```python
from build123d import *

# Parameters (mm, degrees)
F0_W     = 200
F0_H     = 25
F0_H_2   = 5
F1_DEPTH = 5
F2_DEPTH = 13.2
F3_SIZE  = 0.6


with BuildPart() as f1:
    # F0 (on Top) → F1 (new body)
    with BuildSketch(Plane.XY):
        with Locations((100, 12.5)):
            Rectangle(F0_W, F0_H)
        with Locations((100, -2.5)):
            Rectangle(F0_W, F0_H_2)
    extrude(amount=F1_DEPTH)

    # F0 (on Top) → F2 (join)
    with BuildSketch(Plane.XY):
        with Locations((100, -2.5)):
            Rectangle(F0_W, F0_H_2)
    extrude(amount=F2_DEPTH)

    # F3
    f3_edges = [f1.edges().sort_by_distance(p)[0] for p in [
        (100, 25, 5),
        (200, 12.5, 5),
        (200, 25, 2.5),
        (200, 10, 0),
        (200, -5, 6.6),
        (200, -2.5, 13.2),
        (200, 0, 9.1),
        (0, 25, 2.5),
        (100, 25, 0),
        (0, 10, 0),
        (0, 12.5, 5),
        (0, 0, 9.1),
        (0, -2.5, 13.2),
        (0, -5, 6.6),
        (100, 0, 13.2),
        (100, -5, 13.2),
        (100, -5, 0),
    ]]
    chamfer(f3_edges, length=F3_SIZE)


solid = f1.part
```
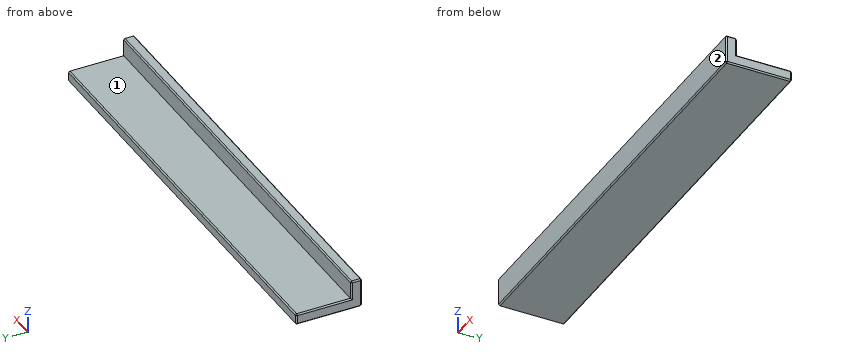
CAD build for the part. Positions are in the model's coordinates, mm. Face numbers are marked on the shaded views. A direction names the side the tool comes from. Round coordinates to 2 decimals unless told otherwise and drop trailing zeros. Order: outer loops, then holes, each group sorted by start corner. A loop starts at its lowest first (then second) coordinate and runs counter-clockwise, first axis right, second up.
Q1. Drop a flat-ended pin along its axis: pin 1 (6 mm diameter, centred on x = 121.5, z = 10, fed in from +Y). Give the stop position or say it passes through.
Q2. Which spindle directions (+Z, -Z, +X, -X, +Y, -Y) get a long thin tool onto all of the face, cutting with end or side? Do the marked faces 1 and 2. Say none if no direction does.
Q3. Slice it at C-C (x = 111). Write the cut outline in (y, z).
Q4. Slice it at B-B (z = 7.5). Write the cut outline in (x, y).
Q5. Slice it at A-A (y = 14.5). Write the cut outline in (x, z).
Q6. Wall check: L1, parallel to Z at x = 158, y = 5.5; L2, parallel to Y at x = 74.5, z = 5.5; L3, parallel to Y at x = 124, z = 4.5. Give the ranges that are in metal, low to high.
Results below:
1. pin 1: stops at y = 0
2. face 1: +Z, +X, -X, +Y
2. face 2: +Z, -Z, +X, -X, -Y
3. outline: (-5, 0.6) - (-4.4, 0) - (24.4, 0) - (25, 0.6) - (25, 4.4) - (24.4, 5) - (0, 5) - (0, 12.6) - (-0.6, 13.2) - (-4.4, 13.2) - (-5, 12.6) - close
4. outline: (0, -4.4) - (0.6, -5) - (199.4, -5) - (200, -4.4) - (200, -0.6) - (199.4, 0) - (0.6, 0) - (0, -0.6) - close
5. outline: (0, 0.6) - (0.6, 0) - (199.4, 0) - (200, 0.6) - (200, 4.4) - (199.4, 5) - (0.6, 5) - (0, 4.4) - close
6. L1: z = 0 to 5
6. L2: y = -5 to 0
6. L3: y = -5 to 24.9
